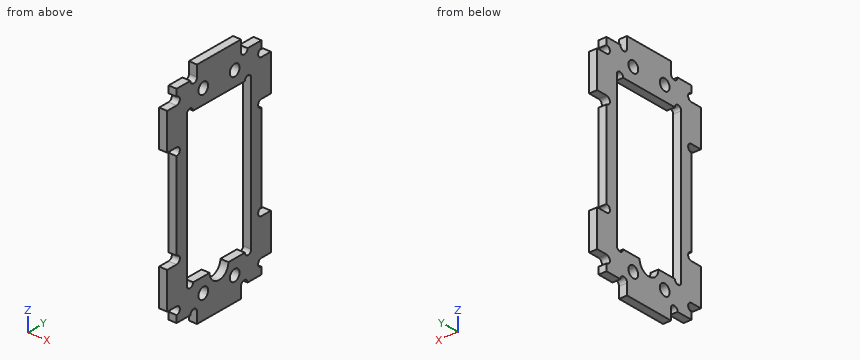
```python
from build123d import *

# Parameters (mm, degrees)
SKETCH_1_R      = 1.55
EXTRUDE_1_DEPTH = 2.2


with BuildPart() as part:
    # 草图1 → 凸台-拉伸1 (new body)
    with BuildSketch(Plane(origin=(0, 0, 0), x_dir=(0, 0, -1), z_dir=(1, 0, 0))):
        with BuildLine():
            Line((-24, 16.5), (-24, 13.5))
            ThreePointArc((-24, 13.5), (-25.05, 12.45), (-26.1, 13.5))
            Line((-26.1, 13.5), (-28, 13.5))
            Line((-28, 13.5), (-28, 9.1))
            ThreePointArc((-28, 9.1), (-27.25753788, 8.79246212), (-26.95, 8.05))
            ThreePointArc((-26.95, 8.05), (-27.25753788, 7.30753788), (-28, 7))
            Line((-28, 7), (-31, 7))
            Line((-31, 7), (-31, -7))
            Line((-31, -7), (-28, -7))
            ThreePointArc((-28, -7), (-27.25753788, -7.30753788), (-26.95, -8.05))
            ThreePointArc((-26.95, -8.05), (-27.25753788, -8.79246212), (-28, -9.1))
            Line((-28, -9.1), (-28, -13.5))
            Line((-28, -13.5), (-26.1, -13.5))
            ThreePointArc((-26.1, -13.5), (-25.05, -12.45), (-24, -13.5))
            Line((-24, -13.5), (-24, -16.5))
            Line((-24, -16.5), (-14, -16.5))
            Line((-14, -16.5), (-14, -13.5))
            ThreePointArc((-14, -13.5), (-12.95, -12.45), (-11.9, -13.5))
            Line((-11.9, -13.5), (11.9, -13.5))
            ThreePointArc((11.9, -13.5), (12.95, -12.45), (14, -13.5))
            Line((14, -13.5), (14, -16.5))
            Line((14, -16.5), (24, -16.5))
            Line((24, -16.5), (24, -13.5))
            ThreePointArc((24, -13.5), (25.05, -12.45), (26.1, -13.5))
            Line((26.1, -13.5), (28, -13.5))
            Line((28, -13.5), (28, -9.1))
            ThreePointArc((28, -9.1), (26.95, -8.05), (28, -7))
            Line((28, -7), (31, -7))
            Line((31, -7), (31, 7))
            Line((31, 7), (28, 7))
            ThreePointArc((28, 7), (26.95, 8.05), (28, 9.1))
            Line((28, 9.1), (28, 13.5))
            Line((28, 13.5), (26.1, 13.5))
            ThreePointArc((26.1, 13.5), (25.05, 12.45), (24, 13.5))
            Line((24, 13.5), (24, 16.5))
            Line((24, 16.5), (14, 16.5))
            Line((14, 16.5), (14, 13.5))
            ThreePointArc((14, 13.5), (12.95, 12.45), (11.9, 13.5))
            Line((11.9, 13.5), (-11.9, 13.5))
            ThreePointArc((-11.9, 13.5), (-12.95, 12.45), (-14, 13.5))
            Line((-14, 13.5), (-14, 16.5))
            Line((-14, 16.5), (-24, 16.5))
        make_face()
        with Locations((-24.5, -5)):
            Circle(SKETCH_1_R, mode=Mode.SUBTRACT)
        with BuildLine():
            Line((20.5, 8.24), (20.5, 3))
            ThreePointArc((20.5, 3), (23.5, 0), (20.5, -3))
            Line((20.5, -3), (20.5, -8.24))
            ThreePointArc((20.5, -8.24), (21.210642315, -8.534357685), (21.505, -9.245))
            ThreePointArc((21.505, -9.245), (21.210642315, -9.955642315), (20.5, -10.25))
            Line((20.5, -10.25), (-20.5, -10.25))
            ThreePointArc((-20.5, -10.25), (-21.505, -9.245), (-20.5, -8.24))
            Line((-20.5, -8.24), (-20.5, 8.24))
            ThreePointArc((-20.5, 8.24), (-21.505, 9.245), (-20.5, 10.25))
            Line((-20.5, 10.25), (20.5, 10.25))
            ThreePointArc((20.5, 10.25), (21.210642315, 9.955642315), (21.505, 9.245))
            ThreePointArc((21.505, 9.245), (21.210642315, 8.534357685), (20.5, 8.24))
        make_face(mode=Mode.SUBTRACT)
        with Locations((24.5, -5)):
            Circle(SKETCH_1_R, mode=Mode.SUBTRACT)
        with Locations((-24.5, 5)):
            Circle(SKETCH_1_R, mode=Mode.SUBTRACT)
        with Locations((24.5, 5)):
            Circle(SKETCH_1_R, mode=Mode.SUBTRACT)
    extrude(amount=EXTRUDE_1_DEPTH)


solid = part.part
```
Verification items for the finished model (mm, model axes). Give positions to 0.01 mm unless a question says otherwise; leave off trailing zeros. Write each loop counter-clockwise with the first axis right and the second up, starting at its lowest first coordinate (ties: lowest second). Pieces come first, ordered by that corner, then holes. Notation, with made-up numbers: (-39.75, 85) - (12.25, 85) arc R21 cw to (12.25, 92) - close; hole circle Ø10 at (-22, 71). An arc over 180 degrees is marked (long way). Put each result on its own line as item: value.
Q1. Scan lines: probe 1 along Y at (x, z) = (0.7, -24.5); probe 2 along Y at (x, z) = (1.3, 16.5); probe 3 along Z at (x, y) = (1, -5.5). Record each from-to range of solid material in increasing order. Write a range as from..to.
Result:
probe 1: -12.61..-6.55, -3.45..3.45, 6.55..12.61
probe 2: -16.5..-10.25, 10.25..16.5
probe 3: -31..-25.97, -23.03..-20.5, 20.5..23.03, 25.97..31
Q2. Depth check by flat-ended pin: P1, Ø1.1, axis at x = 0.5, y = 14.5, coming from the +Z side; P2, Ø1.1, axis at x = 0.5, y = -15.5, coming from the -Z side. Enter the tip coordinate at first touch or a pass-through.
Result:
P1: z = 24
P2: z = -24
Q3. Section check B-B on y = 5. Record the cut outline in (x, z), and give its area (3 significant figures).
Result:
outline: (0, -31) - (2.2, -31) - (2.2, -26.05) - (0, -26.05) - close; (0, -22.95) - (2.2, -22.95) - (2.2, -20.5) - (0, -20.5) - close; (0, 20.5) - (2.2, 20.5) - (2.2, 22.95) - (0, 22.95) - close; (0, 26.05) - (2.2, 26.05) - (2.2, 31) - (0, 31) - close
area: 32.6 mm2
Q4. Section check D-D on x = 0.35. Count the separate pieces of the cut face and the enclosed holes in it, and give its area (3 significant figures).
Result:
separate pieces: 1
enclosed holes: 5
area: 804 mm2
Q5. Section check C-C on z = 1.5. Record the cut outline in (x, y), and give its area (3 significant figures).
Result:
outline: (0, -13.5) - (2.2, -13.5) - (2.2, -10.25) - (0, -10.25) - close; (0, 10.25) - (2.2, 10.25) - (2.2, 13.5) - (0, 13.5) - close
area: 14.3 mm2
Q6. Section check A-A on z = -15.5. Record the cut outline in (x, y).
Result:
outline: (0, -16.5) - (2.2, -16.5) - (2.2, -10.25) - (0, -10.25) - close; (0, 10.25) - (2.2, 10.25) - (2.2, 16.5) - (0, 16.5) - close
